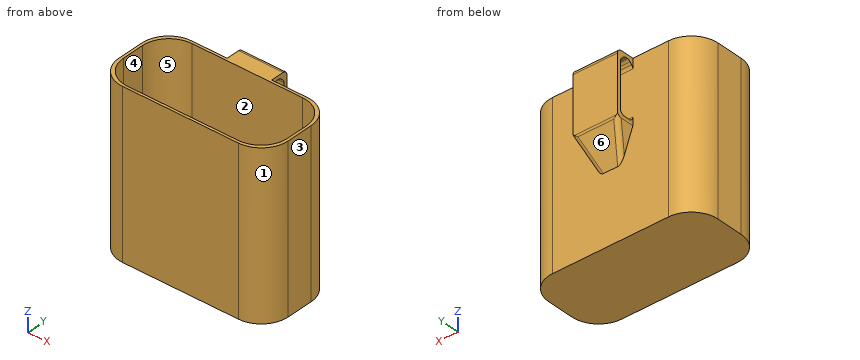
from build123d import *

# Parameters (mm, degrees)
F0_W          = 95
F0_H          = 45
F1_DEPTH      = 1.28
F2_W          = 95
F2_H          = 45
F2_W_2        = 92.12
F2_H_2        = 42.12
F3_DEPTH      = 90
F4_W          = 25
F4_H          = 35
F5_DEPTH      = 10
F6_W          = 8
F6_H          = 31
F7_DEPTH      = 60.001
F9_DEPTH      = 25
F11_DEPTH     = 10
F12_SIZE      = 2.5
F13_T1_DEPTH  = 25
F13_T3_DEPTH  = 37.5
F13_T5_DEPTH  = 28.3493649054
F13_T10_DEPTH = 35.1683904211
F13_T15_DEPTH = 35.1683904211
F14_R         = 15
F15_R         = 15
F16_R         = 15


# Not quite as in the source:
# - a fillet or chamfer that OpenCascade refuses, or shapes differently, is made with other operations: its cross-section is extruded or revolved along the edge and cut away or added


with BuildPart() as f1:
    # F0 (on Top) → F1 (new body)
    with BuildSketch(Plane.XY):
        with Locations((47.5, 22.5)):
            Rectangle(F0_W, F0_H)
    extrude(amount=F1_DEPTH)

    # F2 (on face) → F3 (join)
    with BuildSketch(Plane.XY.offset(1.28)):
        with Locations((47.5, 22.5)):
            Rectangle(F2_W, F2_H)
        with Locations((47.5, 22.5)):
            Rectangle(F2_W_2, F2_H_2, mode=Mode.SUBTRACT)
    extrude(amount=F3_DEPTH)

    # F4 (on face) → F5 (join)
    with BuildSketch(Plane(origin=(0, 45, 0), x_dir=(-1, 0, 0), z_dir=(0, 1, 0))):
        with Locations((-47.5, 73.78)):
            Rectangle(F4_W, F4_H)
    extrude(amount=F5_DEPTH)

    # F6 (on face) → F7 (cut, through all)
    with BuildSketch(Plane.YZ.offset(60)):
        with Locations((49, 73.78)):
            Rectangle(F6_W, F6_H)
    extrude(amount=-F7_DEPTH, mode=Mode.SUBTRACT)

    # F8 (on face) → F9 (join, through all)
    with BuildSketch(Plane.YZ.offset(60)):
        Polygon((55, 56.28), (45, 56.28), (45, 38.9594919243), align=None)
    extrude(amount=-F9_DEPTH)

    # F10 (on face) → F11 (cut, through all)
    with BuildSketch(Plane(origin=(0, 55, 0), x_dir=(-1, 0, 0), z_dir=(0, 1, 0))):
        Polygon((-53.6958506181, 38.9594919243), (-60, 56.28), (-60, 38.9594919243), align=None)
        Polygon((-41.304149382, 38.9594919243), (-35, 38.9594919243), (-35, 56.28), align=None)
    extrude(amount=-F11_DEPTH, mode=Mode.SUBTRACT)

    # F12
    f12_edges = [f1.edges().sort_by_distance(p)[0] for p in [
        (47.5, 45, 89.28),
        (47.5, 53, 89.28),
    ]]
    chamfer(f12_edges, length=F12_SIZE)

    # F13: fillet of radius 2.5 on 10 edges, made by hand

    # F13_s2 → F13_t1 (join)
    with BuildSketch(Plane.YZ.offset(35)):
        with BuildLine():
            ThreePointArc((45, 85.7444660941), (45.1903011687, 86.701174675), (45.732233047, 87.512233047))
            Line((45.732233047, 87.512233047), (45, 86.78))
            Line((45, 86.78), (45, 85.7444660941))
        make_face()
        with BuildLine():
            ThreePointArc((52.267766953, 87.512233047), (52.8096988313, 86.701174675), (53, 85.7444660941))
            Line((53, 85.7444660941), (53, 86.78))
            Line((53, 86.78), (52.267766953, 87.512233047))
        make_face()
        with BuildLine():
            ThreePointArc((50.5, 58.28), (52.267766953, 59.012233047), (53, 60.78))
            Line((53, 60.78), (53, 58.28))
            Line((53, 58.28), (50.5, 58.28))
        make_face()
        with BuildLine():
            ThreePointArc((45, 60.78), (45.732233047, 59.012233047), (47.5, 58.28))
            Line((47.5, 58.28), (45, 58.28))
            Line((45, 58.28), (45, 60.78))
        make_face()
        with BuildLine():
            ThreePointArc((46.767766953, 88.547766953), (47.578825325, 89.0896988313), (48.5355339059, 89.28))
            Line((48.5355339059, 89.28), (47.5, 89.28))
            Line((47.5, 89.28), (46.767766953, 88.547766953))
        make_face()
        with BuildLine():
            ThreePointArc((49.4644660941, 89.28), (50.421174675, 89.0896988313), (51.232233047, 88.547766953))
            Line((51.232233047, 88.547766953), (50.5, 89.28))
            Line((50.5, 89.28), (49.4644660941, 89.28))
        make_face()
    extrude(amount=F13_T1_DEPTH)

    # F13_s4 → F13_t3 (cut)
    with BuildSketch(Plane.YZ.offset(28.75)):
        with BuildLine():
            ThreePointArc((55, 88.78), (54.267766953, 90.547766953), (52.5, 91.28))
            Line((52.5, 91.28), (55, 91.28))
            Line((55, 91.28), (55, 88.78))
        make_face()
    extrude(amount=F13_T3_DEPTH, mode=Mode.SUBTRACT)

    # F13_s6 → F13_t5 (cut)
    with BuildSketch(Plane.YZ.offset(33.3253175473)):
        with BuildLine():
            ThreePointArc((54.6650635095, 55.6998729811), (54.9148145657, 56.3028253683), (55, 56.9498729811))
            Line((55, 56.9498729811), (55, 56.28))
            Line((55, 56.28), (54.6650635095, 55.6998729811))
        make_face()
    extrude(amount=F13_T5_DEPTH, mode=Mode.SUBTRACT)


with BuildPart() as f13_tool8:
    # F13_s9 → F13_t10 (new body)
    with BuildSketch(Plane(origin=(19.397060828, 30.7687201759, 53.2929866286), x_dir=(-0.8459331757, 0.5332889107, 0), z_dir=(0.3006265785, 0.4768709627, 0.8259647361))):
        with BuildLine():
            ThreePointArc((-19.5594103687, -32.1600455029), (-21.2581254439, -32.3827100323), (-22.7013076364, -31.4594345813))
            Line((-22.7013076364, -31.4594345813), (-21.425100455, -33.1315112786))
            Line((-21.425100455, -33.1315112786), (-19.5594103687, -32.1600455029))
        make_face()
    extrude(amount=F13_T10_DEPTH)

    split(bisect_by=Plane.XZ.offset(-45), keep=Keep.BOTTOM)


with BuildPart() as f1_1:
    add(f1.part)

    # F13_t7: cut F13_tool8
    add(f13_tool8.part, mode=Mode.SUBTRACT)


with BuildPart() as f13_tool13:
    # F13_s14 → F13_t15 (new body)
    with BuildSketch(Plane(origin=(-21.3838614404, 33.9202962128, 58.7516764483), x_dir=(0.8459331757, 0.5332889107, 0), z_dir=(0.3006265785, -0.4768709627, -0.8259647361))):
        with BuildLine():
            ThreePointArc((57.6623440552, 10.3859596823), (59.1055262478, 9.4626842314), (60.8042413229, 9.6853487608))
            Line((60.8042413229, 9.6853487608), (58.9385512366, 8.713882985))
            Line((58.9385512366, 8.713882985), (57.6623440552, 10.3859596823))
        make_face()
    extrude(amount=F13_T15_DEPTH)

    split(bisect_by=Plane.XZ.offset(-45), keep=Keep.BOTTOM)


with BuildPart() as f1_2:
    add(f1_1.part)

    # F13_t12: cut F13_tool13
    add(f13_tool13.part, mode=Mode.SUBTRACT)

    # F14
    f14_edges = [f1_2.edges().sort_by_distance(p)[0] for p in [
        (1.44, 43.56, 46.28),
        (1.44, 1.44, 46.28),
        (93.56, 43.56, 46.28),
        (93.56, 1.44, 46.28),
    ]]
    fillet(f14_edges, radius=F14_R)

    # F15
    f15_edges = [f1_2.edges().sort_by_distance(p)[0] for p in [
        (95, 0, 45.64),
        (95, 45, 45.64),
        (0, 45, 45.64),
        (0, 0, 45.64),
    ]]
    fillet(f15_edges, radius=F15_R)

    # F16
    f16_edges = [f1_2.edges().sort_by_distance(p)[0] for p in [
        (47.5, 43.56, 1.28),
        (5.833398, 39.166602, 1.28),
        (89.166602, 39.166602, 1.28),
        (1.44, 22.5, 1.28),
        (93.56, 22.5, 1.28),
        (5.833398, 5.833398, 1.28),
        (89.166602, 5.833398, 1.28),
        (47.5, 1.44, 1.28),
    ]]
    fillet(f16_edges, radius=F16_R)


solid = f1_2.part
Here's how the part is built. I have some questions about the finished solid (model axes, mm). Face numbers are marked on the shaded views. A direction names the side the tool comes from. Round coordinates to 2 decimals unless told otherwise and drop trailing zeros. Order: outer loops, then holes, each group sorted by start corner. A loop starts at its lowest first (then second) coordinate and runs counter-clockwise, first axis right, second up. Notation, with made-up numbers: M 19.5,30 L 46.5,30 A16 cw 46.5,35 Z; hole C 46.5,85.5 d5. An arc over 180 degrees is marked long. Return JSON: item names as keys, results as strings. Group by question number.
1. If we section it at D-D on x = 73: List the corners of the cut face in (y, z) for me, then the cut area to 3 significant figures.
2. Please list where these lines run through material, in increasing order: probe 1 along Y at (x, z) = (27, 72); probe 2 along X at (y, z) = (21, 74); probe 3 along Z at (x, y) = (71, 19).
3. I'm going to push flat-ended pins straight in: pin 1 Ø9.5 at (x, y) = (50.5, 24) entering from +Z; pin 2 Ø5 at (y, z) = (7.5, 18) entering from +X; pin 3 Ø12 at (x, z) = (46.5, 28) entering from +Y. Where does each tip first touch, or does it pass through?
4. If we mould it in two halves opening along Y, with no side actions, what happens to the marked faces 3, 4, 5 and 6? For each: pulls with the +Y half, pulls with the -Y half, needs draft (parallel to the pull), parting line crosses it, or undercut.
5. On a 3-axis mill with a long thin cutter (end or side, diameter ignored), from which of +Z, -Z, +X, -X, +Y, -Y can I reach the whole of each face in a straight line? I mean the marked faces 1 and 2. Say none if no direction works.
6. If we section it at C-C on y = 23: List the corners of the cut face in (x, z) for me.
7. If we section it at B-B on z = 24.5: List the corners of the cut face in (x, y) for me, then the cut area to 3 significant figures.
8. If we section it at A-A on x = 46: List the corners of the cut face in (y, z) for me, then the cut area to 3 significant figures.
Reply:
{
 "1": {"outline": "M 0,0 L 45,0 L 45,91.28 L 43.56,91.28 L 43.56,16.28 A15 cw 28.56,1.28 L 16.44,1.28 A15 cw 1.44,16.28 L 1.44,91.28 L 0,91.28 Z", "area": "413 mm^2"},
 "2": {"probe 1": "0 to 1.44, 43.56 to 45", "probe 2": "0 to 1.44, 93.56 to 95", "probe 3": "0 to 1.28"},
 "3": {"pin 1": "z = 1.28", "pin 2": "x = 94.14", "pin 3": "y = 45"},
 "4": {"face 3": "needs draft", "face 4": "undercut", "face 5": "undercut", "face 6": "pulls with the +Y half"},
 "5": {"face 1": "+Z, -Z, +X, -Y", "face 2": "+Z"},
 "6": {"outline": "M 0,0 L 95,0 L 95,91.28 L 93.56,91.28 L 93.56,16.28 A15 cw 78.56,1.28 L 16.44,1.28 A15 cw 1.44,16.28 L 1.44,91.28 L 0,91.28 Z"},
 "7": {"outline": "M 0,15 A15 ccw 15,0 L 80,0 A15 ccw 95,15 L 95,30 A15 ccw 80,45 L 15,45 A15 ccw 0,30 Z; hole M 1.44,16.44 A15 ccw 16.44,1.44 L 78.56,1.44 A15 ccw 93.56,16.44 L 93.56,28.56 A15 ccw 78.56,43.56 L 16.44,43.56 A15 ccw 1.44,28.56 Z", "area": "395 mm^2"},
 "8": {"outline": "M 0,0 L 45,0 L 45,38.96 L 54.67,55.7 A2.5 ccw 55,56.95 L 55,88.78 A2.5 ccw 52.5,91.28 L 43.56,91.28 L 43.56,16.28 A15 cw 28.56,1.28 L 16.44,1.28 A15 cw 1.44,16.28 L 1.44,91.28 L 0,91.28 Z; hole M 45,60.78 A2.5 ccw 47.5,58.28 L 50.5,58.28 A2.5 ccw 53,60.78 L 53,85.74 A2.5 ccw 52.27,87.51 L 51.23,88.55 A2.5 ccw 49.46,89.28 L 48.54,89.28 A2.5 ccw 46.77,88.55 L 45.73,87.51 A2.5 ccw 45,85.74 Z", "area": "610 mm^2"}
}
